Autodesk Inventor part; units mm, degrees
ref_plane "Начальная плоскость" through (0, 0, 40) normal (0, 0, 1) x (1, 0, 0)
ref_plane "Конечная плоскость" through (0, 0, 200) normal (0, 0, 1) x (1, 0, 0)
ref_plane "РабПлоскость4" through (43.57, 295, 200) normal (0, 0, 1) x (1, 0, 0)
ref_plane "Начальная плоскость" through (0, 0, 40) normal (0, 0, 1) x (1, 0, 0)
ref_plane "Конечная плоскость" through (0, 0, 200) normal (0, 0, 1) x (1, 0, 0)
sketch "Эскиз" plane through (0, 0, 0) normal (0, 0, 1) x (1, 0, 0)
  line L0 (-1.43, 0) -> (-1.43, 40)
  line L1 (-1.43, 40) -> (43.57, 40)
  line L2 (43.57, 40) -> (43.57, 38.1774)
  line L3 (39.9881, 34.1993) -> (11.2338, 31.1771)
  line L4 (4.07, 23.221) -> (4.07, 0)
  line L5 (4.07, 0) -> (-1.43, 0) construction
  line L6 (23.82, 40) -> (23.82, 32.5) construction
  line L7 (43.57, 34.5758) -> (43.57, 32.5) construction
  line L8 (43.57, 32.5) -> (23.82, 32.5) construction
  line L9 (0, 15) -> (0, -27) construction
  line L10 (-5.539, 0) -> (16.0067, 0) construction
  line L11 (-1.43, 0) -> (-1.43, -40)
  line L12 (-1.43, -40) -> (43.57, -40)
  line L13 (43.57, -40) -> (43.57, -38.1774)
  line L14 (39.9881, -34.1993) -> (11.2338, -31.1771)
  line L15 (4.07, -23.221) -> (4.07, 0)
  arc A0 (11.2338, 31.1771) -> (4.07, 23.221) centre (12.07, 23.221) ccw
  arc A1 (4.07, -23.221) -> (11.2338, -31.1771) centre (12.07, -23.221) ccw
  arc A2 (39.9881, 34.1993) -> (43.57, 38.1774) centre (39.57, 38.1774) ccw
  arc A3 (43.57, -38.1774) -> (39.9881, -34.1993) centre (39.57, -38.1774) ccw
  line L16 (0, 56) -> (0, -56) construction
  line L17 (-15.5135, 0) -> (54.308, 0) construction
  point P0 (4.07, 30.4242)
  point P1 (43.57, -34.5758)
  point P2 (4.07, -30.4242)
  point P3 (23.82, -40)
  point P4 (23.82, -32.5)
  dimension "d0" = 5.5
  dimension "d1" = 40
  dimension "d2" = 45
  dimension "d3" = 7.5
  dimension "d4" = 19.75
  dimension "d5" = 2.0758
  dimension "d23" = 8
  dimension "d24" = 4
  dimension "d25" = 1.43
extrude "Тело" add sketch "Эскиз" along normal up to surface (160 mm away) from surface at 40
sketch "Sketch3" plane through (0, 0, 0) normal (0, 0, 1) x (1, 0, 0)
  line L0 (0, 0) -> (10, 0)
ref_plane "Work Plane3" through (0, 0, 0) normal (0, -1, 0) x (1, 0, 0)
sketch "Sketch4" plane through (0, 0, 0) normal (0, -1, 0) x (1, 0, 0)
  line L0 (-2, 40) -> (12, 40)
  line L1 (-2, 200) -> (12, 200)
  dimension "d29" = 160
ref_plane "РабПлоскость4" through (43.57, 295, 200) normal (0, 0, 1) x (1, 0, 0)
split "Разделение1" plane through (43.57, 295, 200) removes the side toward (0, 0, 1)
ref_plane "РабПлоскость5" through (43.57, -375, 40) normal (0, 0, -1) x (-1, 0, 0)
split "Разделение2" plane through (43.57, -375, 40) removes the side toward (0, 0, -1)
equation "\"d0\" = G_T"
equation "\"d1\" = 0.5 * G_H"
equation "\"d2\" = G_W"
equation "\"d3\" = G_T1"
equation "\"d4\" = G_C"
equation "\"d23\" = G_IR"
equation "\"d24\" = G_ER"
equation "\"d25\" = ex"
equation "\"d6\" = G_L"
equation "\"G_W\" = 45"
equation "\"G_T\" = 5.5"
equation "\"G_T1\" = 7.5"
equation "\"G_NG\" = 0.105104"
equation "\"G_ER\" = 4"
equation "\"G_IR\" = 8"
equation "\"G_C\" = 19.75"
equation "\"G_L\" = d29"
equation "\"ex\" = 1.43"
properties part number "ISO 657/11 - CH 80 x 8 - 160" material "Сталь, мягкая"
The listing builds one solid part. Answer for the finished solid, in the listing's coordinates (mm). A direction names the side the tool comes from. Coordinates: 2 decimals unless noted, no trailing zeros. Loops run counter-clockwise (first coordinate to the right, second up) from the corner with the lowest first, then second, coordinate; pieces in that order, holes last. Notation, with made-up numbers: M -36,-9 L -32,-9 A14 ccw -32,1 Z; hole C -36.5,74.5 d2. An arc over 180 degrees is marked long. Answer in a Markdown table with one row per item.
1) Which of the six approach directions +Z, -Z, +X, -X, +Y, -Y give full straight-line access (tool end or side, diameter ignored) to faces 5 (the cylindrical face through (42.57, 35.53, 118.88)), 6 (the flat face through (3, 0, 200))?
Answers below:
| item | result |
|---|---|
| face 5 | +Z, -Z, +X |
| face 6 | +Z, +X, -X, +Y, -Y |
2) Find section C-C (y = -14). Determine the outline of the cut face in (x, z).
Answers below:
| item | result |
|---|---|
| outline | M -1.43,40 L 4.07,40 L 4.07,200 L -1.43,200 Z |
3) Find section D-D (x = 30.5). Determine the outline of the cut face in (y, z), then the cut area to 3 significant figures.
Answers below:
| item | result |
|---|---|
| outline | M -40,40 L -33.2,40 L -33.2,200 L -40,200 Z; M 33.2,40 L 40,40 L 40,200 L 33.2,200 Z |
| area | 2,180 mm^2 |
4) Find the intervals of material crossed by probe 1 along X at (y, z) = (0, 163); probe 2 along Y at (x, z) = (18, 182); probe 3 along Y at (x, z) = (5.5, 131), in increasing order.
Answers below:
| item | result |
|---|---|
| probe 1 | -1.43 to 4.07 |
| probe 2 | -40 to -31.89, 31.89 to 40 |
| probe 3 | -40 to -27.79, 27.79 to 40 |
5) Find section A-A (x = 18.5). Determine the outline of the cut face in (y, z), then the cut area to 3 significant figures.
Answers below:
| item | result |
|---|---|
| outline | M -40,40 L -31.94,40 L -31.94,200 L -40,200 Z; M 31.94,40 L 40,40 L 40,200 L 31.94,200 Z |
| area | 2,580 mm^2 |
6) Given pin 1 (8 mm diameter, centred on y = 18.5, z = 56.5, fed in from +X); pin 2 (5 mm diameter, centred on y = -25.5, z = 92, fed in from +X), each flat-ended and moving along its own axis, determine where each tip first touches the part or whether it passes through.
Answers below:
| item | result |
|---|---|
| pin 1 | x = 4.07 |
| pin 2 | x = 5.65 |
7) Determine the mould class of faces 1 (the flat face through (21, -40, 119)), 2 (the cylindrical face through (6.18, -28.635, 118.88)), 3 (the flat face through (4.07, 0, 119)), 4 (the flat face through (3, 0, 40)) for opening direction Y: released by +Y, released by -Y, zero draft, split by the parting line, or undercut.
Answers below:
| item | result |
|---|---|
| face 1 | released by -Y |
| face 2 | undercut |
| face 3 | undercut |
| face 4 | zero draft |
8) Find section B-B (z = 174). Determine the outline of the cut face in (x, y).
Answers below:
| item | result |
|---|---|
| outline | M -1.43,-40 L 43.57,-40 L 43.57,-38.18 A4 ccw 39.99,-34.2 L 11.23,-31.18 A8 cw 4.07,-23.22 L 4.07,23.22 A8 cw 11.23,31.18 L 39.99,34.2 A4 ccw 43.57,38.18 L 43.57,40 L -1.43,40 Z |
